The model under review builds one solid part; all positions refer to its coordinate system, in mm. A direction names the side the tool comes from. Give positions to 0.01 mm unless a question says otherwise; leave off trailing zeros. Loops run counter-clockwise (first coordinate to the right, second up) from the corner with the lowest first, then second, coordinate; pieces in that order, holes last. Notation, with made-up numbers: M 82.5,49.5 L 102.5,49.5 A27 cw 102.5,88.5 Z; hole C 48,30.5 d6. An arc over 180 degrees is marked long. One line per item, written item: value. Start each with the question number.
Q1. To check wall thickness, follow line 1 along Y through (x, z) = (0, 1.3); line 2 along Z through (x, y) = (-4, 6); line 3 along X through (y, z) = (9, 2.5). State the ranges of each line that lie inside material, in increasing order. Write a range as from..to.
Q2. For pin 1 (2.5 mm diameter, centred on x = -4, z = 2.5, fed in from +Y); pin 2 (4 mm diameter, centred on x = -0.5, y = 9, fed in from -Z), all flat-tipped, find the tip position at first contact; note any pin that passes through.
Q3. We need section D-D on x = -4. Write out the cut boundary in (y, z), plus the area to 3 significant figures.
Q4. We need section A-A on y = -8.75. Write out the cut boundary in (x, z).
Q5. For faces 5 (the face through (-3.194, 7.205, 1.235)), 6 (the face through (0, -11.25, 2)), list the 3-axis set-ups (+Z, -Z, +X, -X, +Y, -Y) from which the entire face can be reached by the end or side of a thin tool; tool diameter is ignored.
Q6. We need section B-B on y = 8.75. Write out the cut boundary in (x, z), plus the area to 3 significant figures.
Q7. We need section C-C on x = 0. Write out the cut boundary in (y, z), plus the area to 3 significant figures.
Q8. Mouldability with a two-part tool opening along X and no side actions: class faces 1 (the face through (-7.75, 0, 2)), 2 (the face through (-4, 3.25, 2)), 3 (the face through (5.43, 7.2, 2.05)), 4 (the face through (0, 0, 5)) as released by +X, released by -X, zero draft, split by the parting line, or undercut.
```python
from build123d import *

# Parameters (mm, degrees)
SKETCH1_W           = 15.5
SKETCH1_H           = 22.5
BOSS_EXTRUDE1_DEPTH = 5
SKETCH2_R           = 1.5
CUT_EXTRUDE1_DEPTH  = 6
SKETCH3_R           = 1.5
CUT_EXTRUDE2_DEPTH  = 8
FILLET1_R           = 0.2
CHAMFER1_SIZE       = 0.2


with BuildPart() as part:
    # Sketch1 → Boss-Extrude1 (new body)
    with BuildSketch(Plane.XY):
        Rectangle(SKETCH1_W, SKETCH1_H)
    extrude(amount=BOSS_EXTRUDE1_DEPTH)

    # Sketch2 → Cut-Extrude1 (cut, through all)
    with BuildSketch(Plane.XY.offset(5)):
        with Locations((0, 8.75)):
            Circle(SKETCH2_R)
        with Locations((0, -8.75)):
            Circle(SKETCH2_R)
    extrude(amount=-CUT_EXTRUDE1_DEPTH, mode=Mode.SUBTRACT)

    # Sketch3 → Cut-Extrude2 (cut)
    with BuildSketch(Plane(origin=(0, 11.25, 0), x_dir=(1, 0, 0), z_dir=(0, 1, 0))):
        with Locations((-4, -2.5)):
            Circle(SKETCH3_R)
        with Locations((4, -2.5)):
            Circle(SKETCH3_R)
    extrude(amount=-CUT_EXTRUDE2_DEPTH, mode=Mode.SUBTRACT)

    # Fillet1
    fillet1_edges = [part.edges().sort_by_distance(p)[0] for p in [
        (-7.75, 0, 5),
        (0, -11.25, 5),
        (7.75, 0, 5),
        (0, -11.25, 0),
        (-7.75, 0, 0),
        (0, 11.25, 0),
        (7.75, 0, 0),
        (0, 11.25, 5),
        (7.75, -11.25, 2.5),
        (-7.75, -11.25, 2.5),
        (-7.75, 11.25, 2.5),
        (7.75, 11.25, 2.5),
    ]]
    fillet(fillet1_edges, radius=FILLET1_R)

    # Chamfer1
    chamfer1_edges = [part.edges().sort_by_distance(p)[0] for p in [
        (-1.5, 8.75, 0),
        (-1.5, 8.75, 5),
        (-1.5, -8.75, 5),
        (-5.5, 11.25, 2.5),
        (2.5, 11.25, 2.5),
    ]]
    chamfer(chamfer1_edges, length=CHAMFER1_SIZE)


solid = part.part
```
Solved:
1. line 1: -11.25..-10.25, -7.25..7.25, 10.25..11.25
1. line 2: 0..1, 4..5
1. line 3: -7.75..-5.5, -2.5..-1.48, 1.48..2.5, 5.5..7.75
2. pin 1: y = 3.25
2. pin 2: z = 0
3. outline: M -11.25,0.2 A0.2 ccw -11.05,0 L 11.05,0 A0.2 ccw 11.25,0.2 L 11.25,0.8 L 11.05,1 L 3.25,1 L 3.25,4 L 11.05,4 L 11.25,4.2 L 11.25,4.8 A0.2 ccw 11.05,5 L -11.05,5 A0.2 ccw -11.25,4.8 Z
3. area: 88.4 mm2
4. outline: M -7.75,0.2 A0.2 ccw -7.55,0 L -1.5,0 L -1.5,4.8 L -1.7,5 L -7.55,5 A0.2 ccw -7.75,4.8 Z; M 1.5,0 L 7.55,0 A0.2 ccw 7.75,0.2 L 7.75,4.8 A0.2 ccw 7.55,5 L 1.7,5 L 1.5,4.8 Z
5. face 5: +Y
5. face 6: +Z, -Z, +X, -X, -Y
6. outline: M -7.75,0.2 A0.2 ccw -7.55,0 L -1.7,0 L -1.5,0.2 L -1.5,4.8 L -1.7,5 L -7.55,5 A0.2 ccw -7.75,4.8 Z; M 1.5,0.2 L 1.7,0 L 7.55,0 A0.2 ccw 7.75,0.2 L 7.75,4.8 A0.2 ccw 7.55,5 L 1.7,5 L 1.5,4.8 Z; hole C -4,2.5 d3; hole C 4,2.5 d3
6. area: 48.2 mm2
7. outline: M -11.25,0.2 A0.2 ccw -11.05,0 L -10.25,0 L -10.25,4.8 L -10.45,5 L -11.05,5 A0.2 ccw -11.25,4.8 Z; M -7.25,0 L 7.05,0 L 7.25,0.2 L 7.25,4.8 L 7.05,5 L -7.05,5 L -7.25,4.8 Z; M 10.25,0.2 L 10.45,0 L 11.05,0 A0.2 ccw 11.25,0.2 L 11.25,4.8 A0.2 ccw 11.05,5 L 10.45,5 L 10.25,4.8 Z
7. area: 82.3 mm2
8. face 1: released by -X
8. face 2: undercut
8. face 3: undercut
8. face 4: zero draft
